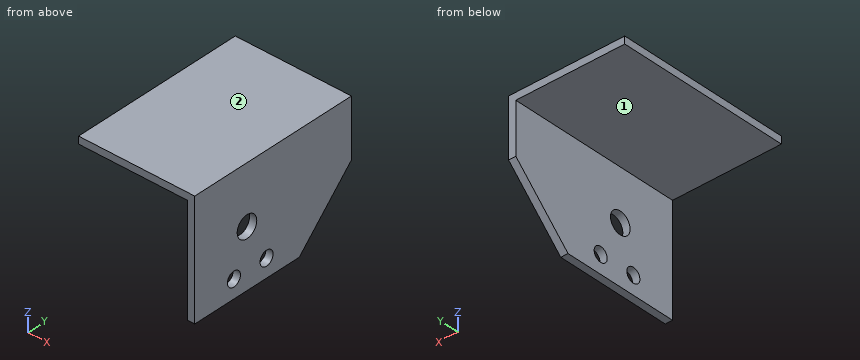
Autodesk Inventor part; units mm, degrees
ref_plane "YZ Plane" through (0, 0, 0) normal (1, 0, 0) x (0, 1, 0)
ref_plane "XZ Plane" through (0, 0, 0) normal (0, 1, 0) x (-1, 0, 0)
ref_plane "XY Plane" through (0, 0, 0) normal (0, 0, 1) x (1, 0, 0)
sketch "Sketch1" plane through (0, 0, 0) normal (0, 1, 0) x (-1, 0, 0)
  line L0 (0, 0) -> (50.8, 0)
  line L1 (50.8, 0) -> (50.8, -3.175)
  line L2 (50.8, -3.175) -> (0, -3.175)
  line L3 (0, -3.175) -> (0, 0)
  line L4 (0, 0) -> (3.175, 0)
  line L5 (3.175, 0) -> (3.175, -50.8)
  line L6 (3.175, -50.8) -> (0, -50.8)
  line L7 (0, -50.8) -> (0, 0)
  dimension "d0" = 50.8
  dimension "d1" = 3.175
  dimension "d2" = 3.175
  dimension "d3" = 50.8
extrude "Extrusion1" add sketch "Sketch1" along normal blind 76.2
sketch "Sketch4" plane through (0, 0, 0) normal (1, 0, 0) x (0, 0, -1)
  line L0 (0, 0) -> (0, 76.2)
  line L1 (0, 0) -> (50.8, 0)
  point P0 (25.4, 25.4)
  dimension "d11" = 25.4
  dimension "d12" = 25.4
hole "Hole1" at (0, 25.4, -25.4) direction (-1, 0, 0) diameter 9.525 end through all
sketch "Sketch5" plane through (-3.175, 0, -50.8) normal (-1, 0, 0) x (0, 0, 1)
  circle A0 centre (25.4, 25.4) radius 4.7625
  line L0 (0, 0) -> (0, 76.2)
  point P0 (50.8, 0)
  point P1 (7.9375, 19.05)
  point P2 (7.9375, 34.925)
  dimension "d20" = 9.525
  dimension "d21" = 6.35
  dimension "d23" = 7.9375
  dimension "d24" = 7.9375
hole "Hole2" at (-3.175, 19.05, -42.8625) at (-3.175, 34.925, -42.8625) direction (1, 0, 0) diameter 6.35 end through all
sketch "Sketch6" plane through (0, 0, 0) normal (1, 0, 0) x (0, 0, -1)
  line L0 (50.8, 0) -> (50.8, 76.2)
  line L1 (50.8, 76.2) -> (25.4, 76.2) construction
  line L2 (50.8, 76.2) -> (3.175, 76.2) construction
  line L3 (25.4, 76.2) -> (50.8, 50.8)
  line L4 (25.4, 76.2) -> (61.321, 76.2) construction
  line L5 (50.8, 50.8) -> (50.8, 76.2)
  line L6 (50.8, 76.2) -> (25.4, 76.2)
  dimension "d32" = 25.4
  dimension "d33" = 45
extrude "Extrusion4" cut sketch "Sketch6" against normal blind 76.2
properties part number "mechanical stop 2x2 angle" material "Aluminum 6061"
Could you check a few things on this model? Use its own coordinates, in mm. Face numbers are marked on the shaded views. A direction names the side the tool comes from. Coordinates: 2 decimals unless noted, no trailing zeros. Order: outer loops, then holes, each group sorted by start corner. A loop starts at its lowest first (then second) coordinate and runs counter-clockwise, first axis right, second up. Notation, with made-up numbers: (-8, 67) - (50, 67) arc R13 ccw to (50, 82) - close; hole circle Ø3 at (68, -9). An arc over 180 degrees is marked (long way). Answer in a Markdown table with one row per item. Add a question column.
(1) If we section it at A-A, the plane y = 25.4: Please give me the cut outline in (x, z) (1 decimal), then the cut area to 3 significant figures.
(2) If we section it at D-D, the plane z = -17: Please give me the cut outline in (x, y) (3 decimals).
(3) I need wall thicknesses on L1, parallel to Y at x = -2.35, z = -25.4; L2, parallel to Z at x = -2, y = 19; L3, parallel to Y at x = -2, z = -25. Which ranges of each line are inside material? Lowest first, please.
(4) If we section it at B-B, the plane z = -28: Please give me the cut outline in (x, y) (3 decimals), then the cut area to 3 significant figures.
(5) Will these pins go through, and if not, where does the flat tip stop? pin 1 (3 mm diameter, centred on x = -13.5, y = 27, fed in from +Z); pin 2 (24 mm diameter, centred on y = 41, z = -37.5, fed in from -X) (3 decimals); pin 3 (4 mm diameter, centred on x = -19.5, y = 34, fed in from -Z) (3 decimals).
(6) On a 3-axis mill with a long thin cutter (end or side, diameter ignored), from which of +Z, -Z, +X, -X, +Y, -Y can I reach the whole of each face in a straight line? I mean the marked faces 1 and 2. Say none if no direction works.
(7) If we section it at C-C, the plane y = 46: Please give me the cut outline in (x, z) (3 decimals), then the cut area to 4 significant figures.
Results are:
| question | item | result |
|---|---|---|
| 1 | outline | (-50.8, -3.2) - (-3.2, -3.2) - (-3.2, -20.6) - (0, -20.6) - (0, 0) - (-50.8, 0) - close; (-3.2, -50.8) - (0, -50.8) - (0, -30.2) - (-3.2, -30.2) - close |
| 1 | area | 282 mm2 |
| 2 | outline | (-3.175, 0) - (0, 0) - (0, 76.2) - (-3.175, 76.2) - close |
| 3 | L1 | y = 0 to 20.64, 30.16 to 76.2 |
| 3 | L2 | z = -50.8 to -46.04, -39.69 to 0 |
| 3 | L3 | y = 0 to 20.65, 30.15 to 76.2 |
| 4 | outline | (-3.175, 0) - (0, 0) - (0, 21.41) - (-3.175, 21.41) - close; (-3.175, 29.39) - (0, 29.39) - (0, 73.6) - (-3.175, 73.6) - close |
| 4 | area | 208 mm2 |
| 5 | pin 1 | stops at z = 0 |
| 5 | pin 2 | stops at x = -3.175 |
| 5 | pin 3 | stops at z = -3.175 |
| 6 | face 1 | -Z, -X, +Y, -Y |
| 6 | face 2 | +Z, +X, -X, +Y, -Y |
| 7 | outline | (-50.8, -3.175) - (-3.175, -3.175) - (-3.175, -50.8) - (0, -50.8) - (0, 0) - (-50.8, 0) - close |
| 7 | area | 312.5 mm2 |
